Could you check a few things on this model? Use its own coordinates, in mm. A direction names the side the tool comes from. Give positions to 0.01 mm unless a question says otherwise; leave off trailing zeros. Order: outer loops, then holes, each group sorted by start corner. A loop starts at its lowest first (then second) coordinate and runs counter-clockwise, first axis right, second up.
(1) Imagine slicing it at C-C, the plane x = 2.5. Write out the boundary of the cut face in (y, z).
(2) On a 3-axis mill with a long thin cutter (end or side, diameter ignored), from which of +Z, -Z, +X, -X, +Y, -Y can I reach the whole of each face in a straight line? I mean faces 1 (the cylindrical face through (54.46, -1.08, -4.88)), 2 (the cylindrical face through (15.46, -1.08, -4.88)), 3 (the flat face through (70, 0, 0)). Say none if no direction works.
(3) Imagine slicing it at A-A, the plane y = 0. State how many separate pieces and enclosed holes the cut face has, then the cut area to 3 significant figures.
(4) Will these pins go through, and if not, where does the flat tip stop? pin 1 (4 mm diameter, centred on x = 2.5, y = 0, fed in from +Z); pin 2 (2 mm diameter, centred on x = 9.5, y = 0.5, fed in from +Z); pin 3 (1 mm diameter, centred on x = 10, y = -4, fed in from +Z).
(5) Imagine slicing it at B-B, the plane x = 32.5. Write out the boundary of the cut face in (y, z), then the cut area to 3 significant figures.
(6) If I drill on probe 1 along X at (y, z) = (0, 2.2); probe 2 along X at (y, z) = (0.5, 3.25); probe 3 along Z at (x, y) = (17.5, 0.25), over which ranges is the centre line in solid material (lowest first)?
from build123d import *

# Parameters (mm, degrees)
SZKIC2_R                        = 1.2
WYTNIJ_WYCI_GNI_CIE1_DEPTH      = 7
WYTNIJ_WYCI_GNI_CIE1_DEPTH_BACK = 7


with BuildPart() as part:
    # Szkic1 → Obrót1 (revolve)
    with BuildSketch(Plane.XY):
        Polygon((0, 0), (70, 0), (70, 2.95), (69, 3.95), (57, 3.95), (57, 5), (52, 5), (52, 6), (18, 6), (18, 5), (13, 5), (13, 3.95), (1, 3.95), (0, 2.95), align=None)
    revolve(axis=Axis((0, 0, 0), (1, 0, 0)))

    # Szkic2 → Wytnij-wyciągnięcie1 (cut, two sides)
    with BuildSketch(Plane.XY) as wytnij_wyci_gni_cie1_sk:
        with Locations((67.5, 0)):
            Circle(SZKIC2_R)
        with Locations((2.5, 0)):
            Circle(SZKIC2_R)
    extrude(amount=WYTNIJ_WYCI_GNI_CIE1_DEPTH, mode=Mode.SUBTRACT)
    extrude(wytnij_wyci_gni_cie1_sk.sketch, amount=-WYTNIJ_WYCI_GNI_CIE1_DEPTH_BACK, mode=Mode.SUBTRACT)


solid = part.part
Answer block:
1. outline: (-1.2, -3.76) - (-1.2, 3.76) arc R3.95 ccw to start; (1.2, -3.76) arc R3.95 ccw to (1.2, 3.76) - close
2. face 1: +X
2. face 2: -X
2. face 3: +Z, -Z, +X, +Y, -Y
3. separate pieces: 3
3. enclosed holes: 0
3. area: 673 mm2
4. pin 1: stops at z = 3.95
4. pin 2: stops at z = 3.95
4. pin 3: stops at z = 1.83
5. outline: circle Ø12 at (0, 0)
5. area: 113 mm2
6. probe 1: x = 0 to 1.3, 3.7 to 66.3, 68.7 to 70
6. probe 2: x = 0.34 to 1.41, 3.59 to 66.41, 68.59 to 69.66
6. probe 3: z = -4.99 to 4.99
